The drawing under review shows one solid part. Ordinate dimensions are in mm from its lowest x, y, z. A direction names the side the tool comes from. Give positions to 0.01 mm unless a question says otherwise; leave off trailing zeros. Write each loop counter-clockwise with the first axis right and the second up, starting at its lowest first coordinate (ties: lowest second). Pieces come first, ordered by that corner, then holes. Notation, with made-up numbers: M 80,33 L 130,33 A32 cw 130,60 Z; hole C -10.75,-22 d8. An arc over 180 degrees is marked long. Use one line per item in the form item = value. Start each with the question number.
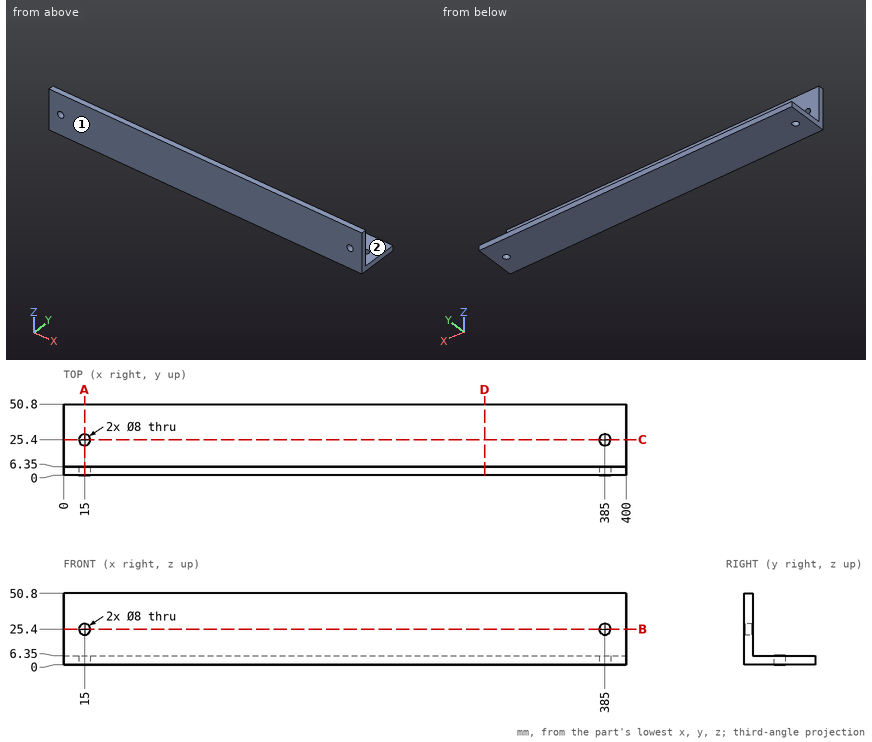
1. For the marked faces 1 and 2, list the 3-axis set-ups (+Z, -Z, +X, -X, +Y, -Y) from which the entire face can be reached by the end or side of a thin tool; tool diameter is ignored.
2. We need section B-B (z = 25.4). State the section outline as (x, y) points, and give its area (3 significant figures).
3. We need section A-A (x = 15). State the section outline as (y, z) points.
4. We need section D-D (x = 299.5). State the section outline as (y, z) points, and give its area (3 significant figures).
5. To check wall thickness, follow L1, parallel to X at y = 1.5, z = 25.4; L2, parallel to Z at x = 385, y = 3.25; L3, parallel to Z at x = 236.5, y = 30. State the ranges of each line that lie inside material, in increasing order.
6. Clearance check with flat-ended pins moving along their axes: pin 1 Ø13 at (x, y) = (15, 25.4) entering from +Z; pin 2 Ø5 at (x, z) = (62, 29) entering from +Y. State where each tip first meets the part, or that it passes through.
Answer block:
q1.face_1 = +Z, -Z, +X, -X, -Y
q1.face_2 = +Z, +X, -X, +Y
q2.outline = M 0,0 L 11,0 L 11,6.35 L 0,6.35 Z; M 19,0 L 381,0 L 381,6.35 L 19,6.35 Z; M 389,0 L 400,0 L 400,6.35 L 389,6.35 Z
q2.area = 2,440 mm^2
q3.outline = M 0,0 L 21.4,0 L 21.4,6.35 L 6.35,6.35 L 6.35,21.4 L 0,21.4 Z; M 0,29.4 L 6.35,29.4 L 6.35,50.8 L 0,50.8 Z; M 29.4,0 L 50.8,0 L 50.8,6.35 L 29.4,6.35 Z
q4.outline = M 0,0 L 50.8,0 L 50.8,6.35 L 6.35,6.35 L 6.35,50.8 L 0,50.8 Z
q4.area = 605 mm^2
q5.L1 = 0 to 11, 19 to 381, 389 to 400
q5.L2 = 0 to 21.4, 29.4 to 50.8
q5.L3 = 0 to 6.35
q6.pin_1 = 6.35
q6.pin_2 = 6.35
